from build123d import *

# Parameters (mm, degrees)
SKETCH1_R           = 22.225
SKETCH1_R_2         = 13.8684
BOSS_EXTRUDE1_DEPTH = 17.018
SKETCH1_3_R         = 19.05
SKETCH1_3_R_2       = 11.8872
BOSS_EXTRUDE2_DEPTH = 15.748
BOSS_EXTRUDE3_DEPTH = 3.175
SKETCH3_W           = 68.65982448
SKETCH3_H           = 6.35
BOSS_EXTRUDE5_DEPTH = 10.795


with BuildPart() as part:
    # Sketch1 → Boss-Extrude1 (new, symmetric)
    with BuildSketch(Plane.XY):
        with Locations((-50.8, 0)):
            Circle(SKETCH1_R)
        with Locations((-50.8, 0)):
            Circle(SKETCH1_R_2, mode=Mode.SUBTRACT)
    extrude(amount=BOSS_EXTRUDE1_DEPTH, both=True)



with BuildPart() as body_2:
    # Sketch1_3 → Boss-Extrude2 (new, symmetric)
    with BuildSketch(Plane.XY):
        with Locations((50.8, 0)):
            Circle(SKETCH1_3_R)
        with Locations((50.8, 0)):
            Circle(SKETCH1_3_R_2, mode=Mode.SUBTRACT)
    extrude(amount=BOSS_EXTRUDE2_DEPTH, both=True)


with BuildPart() as part_1:
    add(part.part)

    add(body_2.part)  # Boss-Extrude3 merges body 2
    # Sketch1_4 → Boss-Extrude3 (add, symmetric)
    with BuildSketch(Plane.XY):
        with BuildLine():
            Line((40.080718494, 15.748), (-35.117171142, 15.748))
            ThreePointArc((-35.117171142, 15.748), (-30.275606021, 8.526422275), (-28.575, 0))
            ThreePointArc((-28.575, 0), (-30.275606021, -8.526422275), (-35.117171142, -15.748))
            Line((-35.117171142, -15.748), (40.080718494, -15.748))
            ThreePointArc((40.080718494, -15.748), (31.75, 0), (40.080718494, 15.748))
        make_face()
    extrude(amount=BOSS_EXTRUDE3_DEPTH, both=True)

    # Sketch3 → Boss-Extrude5 (add, symmetric)
    with BuildSketch(Plane.XY):
        Rectangle(SKETCH3_W, SKETCH3_H)
    extrude(amount=BOSS_EXTRUDE5_DEPTH, both=True)


solid = part_1.part
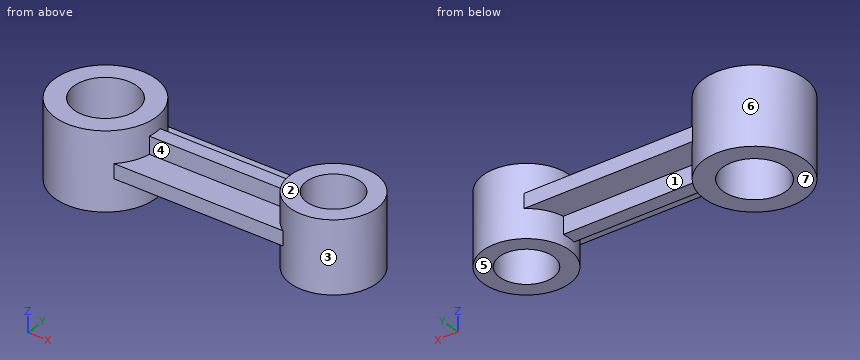
Source: CAD feature listing. Evaluate the final solid. Frame: model axes, mm. Face numbers are marked on the shaded views. A direction names the side the tool comes from. Round coordinates to 2 decimals unless told otherwise and drop trailing zeros. Loops run counter-clockwise (first coordinate to the right, second up) from the corner with the lowest first, then second, coordinate; pieces in that order, holes last. Notation, with made-up numbers: (23.25, -3.5) -> (65.25, -3.5) arc R20 cw to (65.25, 35.5) -> close; hole circle Ø7 at (-40, 27). An arc over 180 degrees is marked (long way). Answer as a JSON object with one key per item and string values. Group by question number.
Q1. Mould query, pull axis X, two halves, no side actions, for the marked faces 6 and 7. Classes: pulls with the +X half, pulls with the -X half, needs draft (parallel to the pull), parting line crosses it, or undercut.
Q2. Ray query, line 1 (Y direction, x = -50.8, z = 7.5) (3 decimals); line 2 (X direction, y = -6.5, z = 11.5); line 3 (X direction, y = 2, z = -1). Return the intervals inside material, ascending. Write a range as from..to.
Q3. Access query for the marked faces 1, 2, 3, 4 and 5. Directions: +Z, -Z, +X, -X, +Y, -Y. A direction counts if a zero-diameter tool reaches every point of the face in a straight line with its end or side. Return the directions, or none.
Q4. Section query B-B (y = 0). Output: boundary loops of the cut face in (x, z) (3 decimals), plus the area to 3 significant figures.
Q5. Section query D-D (z = 1). Output: boundary loops of the cut face in (x, y) (3 decimals).
Q6. Section query C-C (z = -12.5). Output: boundary loops of the cut face in (x, y) (3 decimals), plus the area to 3 significant figures.
Q7. Contact query for flat-ended pins moving along their axis: P1, Ø6, axis at x = 6.5, z = 7.5, coming from the -Y side (3 decimals); P2, Ø10, axis at y = 7, z = 6.5, coming from the -X side; P3, Ø10, axis at x = -15, y = 11.5, coming from the +Z side (3 decimals); P4, Ø5, axis at y = 0.5, z = -11, coming from the +X side. Output: stop coordinate, or through.
Q8. Section query A-A (x = -50.8). Output: boundary loops of the cut face in (y, z) (3 decimals).
Completed:
{
 "1": {"face 6": "undercut", "face 7": "needs draft"},
 "2": {"line 1": "-22.225..-13.868, 13.868..22.225", "line 2": "-72.05..-63.05, -38.55..-29.55, 32.89..40.85, 60.75..68.71", "line 3": "-72.93..-64.52, -37.08..39.08, 62.52..69.74"},
 "3": {"face 1": "-Z, +Y", "face 2": "+Z, +X, +Y, -Y", "face 3": "none", "face 4": "+Z, -Y", "face 5": "-Z, +X, +Y, -Y"},
 "4": {"outline": "(-73.025, -17.018) -> (-64.668, -17.018) -> (-64.668, 17.018) -> (-73.025, 17.018) -> close; (-36.932, -17.018) -> (-28.575, -17.018) -> (-28.575, -10.795) -> (31.75, -10.795) -> (31.75, -15.748) -> (38.913, -15.748) -> (38.913, 15.748) -> (31.75, 15.748) -> (31.75, 10.795) -> (-28.575, 10.795) -> (-28.575, 17.018) -> (-36.932, 17.018) -> close; (62.687, -15.748) -> (69.85, -15.748) -> (69.85, 15.748) -> (62.687, 15.748) -> close", "area": "2,320 mm²"},
 "5": {"outline": "(-35.117, -15.748) -> (40.081, -15.748) arc R19.05 ccw (long way) to (40.081, 15.748) -> (-35.117, 15.748) arc R22.225 ccw (long way) to start; hole circle Ø27.737 at (-50.8, 0); hole circle Ø23.774 at (50.8, 0)"},
 "6": {"outline": "circle Ø44.45 at (-50.8, 0); circle Ø38.1 at (50.8, 0); hole circle Ø27.737 at (-50.8, 0); hole circle Ø23.774 at (50.8, 0)", "area": "1,640 mm²"},
 "7": {"P1": "y = -3.175", "P2": "x = -72.93", "P3": "z = 3.175", "P4": "x = 69.85"},
 "8": {"outline": "(-22.225, -17.018) -> (-13.868, -17.018) -> (-13.868, 17.018) -> (-22.225, 17.018) -> close; (13.868, -17.018) -> (22.225, -17.018) -> (22.225, 17.018) -> (13.868, 17.018) -> close"}
}
